```python
from build123d import *

# Parameters (mm, degrees)
SKETCH1_W                    = 13.5
SKETCH1_H                    = 90
BOSS_EXTRUDE1_DEPTH          = 10
F_1_4_28_TAPPED_HOLE1_D      = 5.4102
F_5_0_5_DIAMETER_HOLE1_D     = 5
F_5_0_5_DIAMETER_HOLE1_DEPTH = 49.5
F_5_0_5_DIAMETER_HOLE1_TIP   = 1.502151548
CUT_EXTRUDE2_DEPTH           = 5


with BuildPart() as part:
    # Sketch1 → Boss-Extrude1 (new body)
    with BuildSketch(Plane(origin=(0, 0, 0), x_dir=(0, 0, -1), z_dir=(1, 0, 0))):
        with Locations((1.965094474, 8.62782)):
            Rectangle(SKETCH1_W, SKETCH1_H)
    extrude(amount=BOSS_EXTRUDE1_DEPTH)

    # 1/4-28 Tapped Hole1 (through all)
    with Locations(Plane(origin=(10, 0, 0), x_dir=(0, 0, -1), z_dir=(1, 0, 0))):
        with Locations((1.965094474, 25.62782), (1.965094474, -8.37218)):
            Hole(F_1_4_28_TAPPED_HOLE1_D / 2)

    # Ø5.0 (5) Diameter Hole1
    with Locations(Plane(origin=(10, 0, 0), x_dir=(0, 0, -1), z_dir=(1, 0, 0))):
        with Locations((1.965094474, 42.62782), (1.965094474, -25.37218), (1.965094474, 8.62782)):
            Hole(F_5_0_5_DIAMETER_HOLE1_D / 2, depth=F_5_0_5_DIAMETER_HOLE1_DEPTH)
            with Locations((0, 0, -(F_5_0_5_DIAMETER_HOLE1_DEPTH + F_5_0_5_DIAMETER_HOLE1_TIP / 2))):  # 118° drill point
                Cone(0, F_5_0_5_DIAMETER_HOLE1_D / 2, F_5_0_5_DIAMETER_HOLE1_TIP, mode=Mode.SUBTRACT)

    # Sketch7 → Cut-Extrude2 (cut)
    with BuildSketch(Plane.ZY):
        Polygon((2.009905526, 40.33285268), (2.009905526, 44.92278732), (-1.965094474, 47.21775464), (-5.940094474, 44.92278732), (-5.940094474, 40.33285268), (-1.965094474, 38.03788536), align=None)
        Polygon((2.009905526, 6.33285268), (2.009905526, 10.92278732), (-1.965094474, 13.21775464), (-5.940094474, 10.92278732), (-5.940094474, 6.33285268), (-1.965094474, 4.03788536), align=None)
        Polygon((2.009905526, -27.66714732), (2.009905526, -23.07721268), (-1.965094474, -20.78224536), (-5.940094474, -23.07721268), (-5.940094474, -27.66714732), (-1.965094474, -29.96211464), align=None)
    extrude(amount=-CUT_EXTRUDE2_DEPTH, mode=Mode.SUBTRACT)


solid = part.part
```
Input: part model. Units: mm. Frame: model coordinates. A direction names the side the tool comes from. Coordinates: 2 decimals unless noted, no trailing zeros. Loops run counter-clockwise (first coordinate to the right, second up) from the corner with the lowest first, then second, coordinate; pieces in that order, holes last. Notation, with made-up numbers: M -4,37.5 L 36,37.5 A30 ccw 36,61.5 Z; hole C 67,67 d8. An arc over 180 degrees is marked long. Answer in a Markdown table with one row per item.
1. Section B-B, the plane z = -3.25. Count the separate pieces of the cut face and the enclosed holes in it, then the cut area to 3 significant figures.
Response:
| item | result |
|---|---|
| separate pieces | 6 |
| enclosed holes | 0 |
| area | 625 mm2 |
2. Section C-C, the plane x = 3. Output: boundary loops of the cut face in (y, z).
Response:
| item | result |
|---|---|
| outline | M -36.37,-8.72 L 53.63,-8.72 L 53.63,4.78 L -36.37,4.78 Z; hole M -29.96,-1.97 L -27.67,-5.94 L -23.08,-5.94 L -20.78,-1.97 L -23.08,2.01 L -27.67,2.01 Z; hole C -8.37,-1.97 d5.41; hole M 4.04,-1.97 L 6.33,-5.94 L 10.92,-5.94 L 13.22,-1.97 L 10.92,2.01 L 6.33,2.01 Z; hole C 25.63,-1.97 d5.41; hole M 38.04,-1.97 L 40.33,-5.94 L 44.92,-5.94 L 47.22,-1.97 L 44.92,2.01 L 40.33,2.01 Z |
3. Section A-A, the plane x = 8.5. Output: boundary loops of the cut face in (y, z).
Response:
| item | result |
|---|---|
| outline | M -36.37,-8.72 L 53.63,-8.72 L 53.63,4.78 L -36.37,4.78 Z; hole C -25.37,-1.97 d5; hole C -8.37,-1.97 d5.41; hole C 8.63,-1.97 d5; hole C 25.63,-1.97 d5.41; hole C 42.63,-1.97 d5 |
4. Reachability of faces 4 (the cylindrical face through (4.9, -11, -2.6)), 5 (the flat face through (5, 40.7, -3.8)) from +Z, -Z, +X, -X, +Y, -Y: full face, straight path, thin tool, end or side. Return the list, or none.
Response:
| item | result |
|---|---|
| face 4 | +X, -X |
| face 5 | -X |
5. Draft query along Z for faces 1 (the flat face through (5, 6.7, -3.8)), 2 (the flat face through (5, 8, -8.715)), 3 (the flat face through (10, 9, -5)). Return one class per face: pulls with the +Z half, pulls with the -Z half, needs draft (parallel to the pull), parting line crosses it, or undercut.
Response:
| item | result |
|---|---|
| face 1 | undercut |
| face 2 | pulls with the -Z half |
| face 3 | needs draft |
6. First-contact query: pin 1 (4 mm diameter, centred on y = 8.63, z = -1.97, fed in from +X); pin 2 (4 mm diameter, centred on y = -25.5, z = -2.5, fed in from -X); pin 3 (7 mm diameter, centred on y = -8.37, z = -1.97, fed in from +X). Flat tips, straight axial feed; report the tip coordinate or a pass-through.
Response:
| item | result |
|---|---|
| pin 1 | passes through |
| pin 2 | stops at x = 5 |
| pin 3 | stops at x = 10 |
7. Material intervals for line 1 (Z direction, x = 4.25, y = 6.5); line 2 (Y direction, x = 1.5, z = 0.25); line 3 (Y direction, x = 1, z = -3.5), sorted ascending.
Response:
| item | result |
|---|---|
| line 1 | z = -8.72 to -5.94, 2.01 to 4.78 |
| line 2 | y = -36.37 to -28.68, -22.06 to -9.92, -6.82 to 5.32, 11.94 to 24.08, 27.18 to 39.32, 45.94 to 53.63 |
| line 3 | y = -36.37 to -29.08, -21.67 to -10.6, -6.14 to 4.92, 12.33 to 23.4, 27.86 to 38.92, 46.33 to 53.63 |
